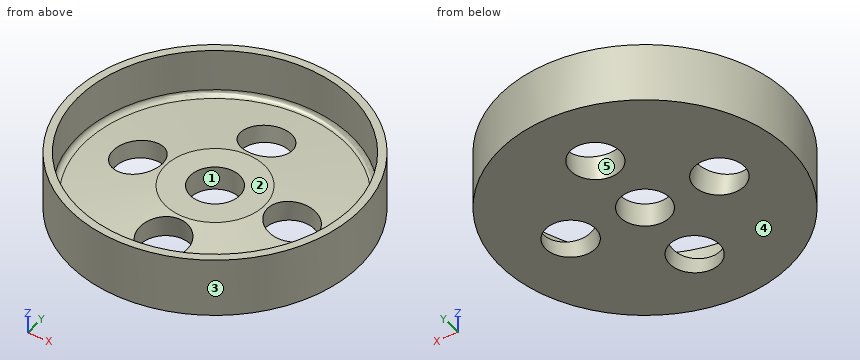
from build123d import *

# Parameters (mm, degrees)
F2_R            = 5
F3_DEPTH        = 4.8063913105
F5_R            = 5
F6_DEPTH        = 4.7469386033
F6_COPIES_COUNT = 4


# Not quite as in the source:
# - a pattern or mirror of a feature is missing from the dataset's text; its kind, count and spacing are read off the source's solid


with BuildPart() as f1:
    # F0 (on Right) → F1 (revolve)
    with BuildSketch(Plane.YZ):
        with BuildLine():
            Line((0, 0), (0, 4.8063913105))
            Line((0, 4.8063913105), (-10, 4.8063913105))
            Line((-10, 4.8063913105), (-26.410826899, 2.5))
            ThreePointArc((-26.410826899, 2.5), (-27.206059029, 2.7355584885), (-27.55, 3.4902680687))
            Line((-27.55, 3.4902680687), (-27.55, 12))
            Line((-27.55, 12), (-29.15, 12))
            Line((-29.15, 12), (-29.15, 0))
            Line((-29.15, 0), (0, 0))
        make_face()
    revolve(axis=Axis((0, 0, 11.0792994889), (0, 0, 1)))

    # F2 (on face) → F3 (cut, through all)
    with BuildSketch(Plane(origin=(0, 0, 0), x_dir=(1, 0, 0), z_dir=(0, 0, -1))):
        Circle(F2_R)
    extrude(amount=-F3_DEPTH, mode=Mode.SUBTRACT)

    # F5 (on line) → F6 (cut, through all)
    with BuildSketch(Plane(origin=(0, -0.8561020162, 6.0914823656), x_dir=(1, 0, 0), z_dir=(0, -0.139173101, 0.9902680687))):
        with Locations((0, -15)):
            Circle(F5_R)
    f6 = extrude(amount=-F6_DEPTH, mode=Mode.SUBTRACT)

    # F6_copies: F6 ×4 about axis
    f6_copies_axis = Axis((0, 0, 0), (0, 0, 1))
    for i in range(1, F6_COPIES_COUNT):
        add(f6.rotate(f6_copies_axis, i * 360 / F6_COPIES_COUNT), mode=Mode.SUBTRACT)


solid = f1.part
Source: CAD feature listing. Evaluate the final solid. Frame: model axes, mm. Face numbers are marked on the shaded views. A direction names the side the tool comes from. Coordinates: 2 decimals unless noted, no trailing zeros. Loops run counter-clockwise (first coordinate to the right, second up) from the corner with the lowest first, then second, coordinate; pieces in that order, holes last. Notation, with made-up numbers: (87.25, -25.5) - (122.25, -25.5) arc R17 cw to (122.25, -8.5) - close; hole circle Ø10 at (34, -18.5). An arc over 180 degrees is marked (long way). One line per question, with ' | ' between items.
1) Pull-direction query (X, two-part tool) for the marked faces 3, 4 and 5; classes: released by +X, released by -X, zero draft, split by the parting line, or undercut.
Report:
face 3: split by the parting line | face 4: zero draft | face 5: undercut
2) Section A-A, the plane y = 0. Return loops of the section in (x, z), then the cut area to 3 significant figures.
Report:
outline: (-29.15, 0) - (-20.2, 0) - (-20.66, 3.31) - (-26.41, 2.5) arc R1 cw to (-27.55, 3.49) - (-27.55, 12) - (-29.15, 12) - close; (-10.76, 4.7) - (-10.1, 0) - (-5, 0) - (-5, 4.81) - (-10, 4.81) - close; (5, 0) - (10.1, 0) - (10.76, 4.7) - (10, 4.81) - (5, 4.81) - close; (20.2, 0) - (29.15, 0) - (29.15, 12) - (27.55, 12) - (27.55, 3.49) arc R1 cw to (26.41, 2.5) - (20.66, 3.31) - close | area: 132 mm²
3) Set-up query: the marked faces 1 and 2. Return all of +Z, -Z, +X, -X, +Y, -Y with unobstructed straight access to the full face (end or side cutting, diameter ignored); none if empty.
Report:
face 1: +Z, -Z | face 2: +Z
4) First-contact query: P1, Ø4, axis at x = 6.5, z = 3.5, coming from the -Y side; P2, Ø6, axis at y = -11, z = 7.5, coming from the +X side; P3, Ø2, axis at x = -16.5, z = 5.5, coming from the +Y side; P4, Ø4, axis at x = 14, y = -21, coming from the -Z side. Flat tips, straight axial feed; report the tip coordinate or a pass-through.
Report:
P1: stops at y = -28.8 | P2: stops at x = 28.03 | P3: stops at y = 24.69 | P4: stops at z = 0
5) Section C-C, the plane z = 10. Return loops of the section in (x, y), then the cut area to 3 significant figures.
Report:
outline: circle Ø58.3 at (0, 0); hole circle Ø55.1 at (0, 0) | area: 285 mm²
6) Line query: line 1 along X through (y, z) = (0, 2); line 2 along X through (y, z) = (0, 1); line 3 along X through (y, z) = (0, 10.25). Output: solid intervals per line, ascending.
Report:
line 1: x = -29.15 to -20.48, -10.38 to -5, 5 to 10.38, 20.48 to 29.15 | line 2: x = -29.15 to -20.34, -10.24 to -5, 5 to 10.24, 20.34 to 29.15 | line 3: x = -29.15 to -27.55, 27.55 to 29.15
